Could you check a few things on this model? Use its own coordinates, in mm. A direction names the side the tool comes from. Round coordinates to 2 decimals unless told otherwise and drop trailing zeros. Loops run counter-clockwise (first coordinate to the right, second up) from the corner with the lowest first, then second, coordinate; pieces in that order, holes last. Notation, with made-up numbers: (-2.75, 64.25) -> (21.25, 64.25) arc R28 cw to (21.25, 83.25) -> close; hole circle Ø6 at (-28, -32). An arc over 180 degrees is marked (long way). One line per item, written item: value.
from build123d import *

# Parameters (mm, degrees)
F1_DEPTH = 11
F2_DEPTH = 4
F3_DEPTH = 10
F4_DEPTH = 5
F5_R     = 2


# Not quite as in the source:
# - a feature names something its author has since deleted; it is built from what else it names


with BuildPart() as f1:
    # F0 (on Top) → F1 (new body)
    with BuildSketch(Plane.XY):
        with BuildLine():
            ThreePointArc((93, 77.5), (92.267766953, 79.267766953), (90.5, 80))
            Line((90.5, 80), (37, 80))
            Line((37, 80), (25, 80))
            Line((25, 80), (19, 80))
            Line((19, 80), (-7, 80))
            Line((-7, 80), (-13, 80))
            Line((-13, 80), (-25, 80))
            Line((-25, 80), (-74, 80))
            Line((-74, 80), (-91.5, 80))
            ThreePointArc((-91.5, 80), (-93.267766953, 79.267766953), (-94, 77.5))
            Line((-94, 77.5), (-94, 76))
            Line((-94, 76), (-94, 0))
            Line((-94, 0), (-94, -1.5))
            ThreePointArc((-94, -1.5), (-93.267766953, -3.267766953), (-91.5, -4))
            Line((-91.5, -4), (-88, -4))
            Line((-88, -4), (-86, -4))
            Line((-86, -4), (-71, -4))
            Line((-71, -4), (-28.6959191337, -4))
            Line((-28.6959191337, -4), (67.7072161436, -4))
            Line((67.7072161436, -4), (88, -4))
            Line((88, -4), (90.5, -4))
            ThreePointArc((90.5, -4), (92.267766953, -3.267766953), (93, -1.5))
            Line((93, -1.5), (93, 0))
            Line((93, 0), (93, 76))
            Line((93, 76), (93, 77.5))
        make_face()
        with BuildLine():
            ThreePointArc((90, 2.5), (89.267766953, 0.732233047), (87.5, 0))
            Line((87.5, 0), (-87.5, 0))
            ThreePointArc((-87.5, 0), (-89.267766953, 0.732233047), (-90, 2.5))
            Line((-90, 2.5), (-90, 73.5))
            ThreePointArc((-90, 73.5), (-89.267766953, 75.267766953), (-87.5, 76))
            Line((-87.5, 76), (87.5, 76))
            ThreePointArc((87.5, 76), (89.267766953, 75.267766953), (90, 73.5))
            Line((90, 73.5), (90, 2.5))
        make_face(mode=Mode.SUBTRACT)
    extrude(amount=F1_DEPTH)

    # F0 (on Top) → F2 (join)
    with BuildSketch(Plane.XY):
        with BuildLine():
            Line((-87.5, 0), (87.5, 0))
            ThreePointArc((87.5, 0), (89.267766953, 0.732233047), (90, 2.5))
            Line((90, 2.5), (90, 73.5))
            ThreePointArc((90, 73.5), (89.267766953, 75.267766953), (87.5, 76))
            Line((87.5, 76), (-87.5, 76))
            ThreePointArc((-87.5, 76), (-89.267766953, 75.267766953), (-90, 73.5))
            Line((-90, 73.5), (-90, 2.5))
            ThreePointArc((-90, 2.5), (-89.267766953, 0.732233047), (-87.5, 0))
        make_face()
        with BuildLine():
            Line((-77.5, 66), (77.5, 66))
            ThreePointArc((77.5, 66), (79.267766953, 65.267766953), (80, 63.5))
            Line((80, 63.5), (80, 12.5))
            ThreePointArc((80, 12.5), (79.267766953, 10.732233047), (77.5, 10))
            Line((77.5, 10), (-77.5, 10))
            ThreePointArc((-77.5, 10), (-79.267766953, 10.732233047), (-80, 12.5))
            Line((-80, 12.5), (-80, 63.5))
            ThreePointArc((-80, 63.5), (-79.267766953, 65.267766953), (-77.5, 66))
        make_face(mode=Mode.SUBTRACT)
        with BuildLine():
            Line((-25, 80), (-13, 80))
            Line((-13, 80), (-13, 89.5))
            ThreePointArc((-13, 89.5), (-13.732233047, 91.267766953), (-15.5, 92))
            Line((-15.5, 92), (-22.5, 92))
            ThreePointArc((-22.5, 92), (-24.267766953, 91.267766953), (-25, 89.5))
            Line((-25, 89.5), (-25, 80))
        make_face()
        with BuildLine():
            Line((-7, 80), (19, 80))
            Line((19, 80), (19, 89.5))
            ThreePointArc((19, 89.5), (18.267766953, 91.267766953), (16.5, 92))
            Line((16.5, 92), (-4.5, 92))
            ThreePointArc((-4.5, 92), (-6.267766953, 91.267766953), (-7, 89.5))
            Line((-7, 89.5), (-7, 80))
        make_face()
        with BuildLine():
            Line((25, 80), (37, 80))
            Line((37, 80), (37, 89.5))
            ThreePointArc((37, 89.5), (36.267766953, 91.267766953), (34.5, 92))
            Line((34.5, 92), (27.5, 92))
            ThreePointArc((27.5, 92), (25.732233047, 91.267766953), (25, 89.5))
            Line((25, 89.5), (25, 80))
        make_face()
    extrude(amount=F2_DEPTH)

    # F0 (on Top) → F3 (join)
    with BuildSketch(Plane.XY):
        with BuildLine():
            Line((93, -81.5), (93, -1.5))
            ThreePointArc((93, -1.5), (92.267766953, -3.267766953), (90.5, -4))
            Line((90.5, -4), (88, -4))
            Line((88, -4), (67.7072161436, -4))
            ThreePointArc((67.7072161436, -4), (74.7782839555, -6.9289321881), (77.7072161436, -14))
            Line((77.7072161436, -14), (77.7072161436, -58.7379819401))
            ThreePointArc((77.7072161436, -58.7379819401), (73.0879609173, -67.1669549309), (63.4976990076, -67.8088124137))
            Line((63.4976990076, -67.8088124137), (-32.9054362697, -23.0708304737))
            ThreePointArc((-32.9054362697, -23.0708304737), (-38.4608642113, -11.8445771571), (-28.6959191337, -4))
            Line((-28.6959191337, -4), (-71, -4))
            Line((-71, -4), (-71, -10.9733034172))
            Line((-71, -10.9733034172), (-64.3552474564, -14.0623617917))
            Line((-64.3552474564, -14.0623617917), (80.7072161436, -81.5))
            Line((80.7072161436, -81.5), (93, -81.5))
        make_face()
    extrude(amount=F3_DEPTH)

    # F0 (on Top) → F4 (join)
    with BuildSketch(Plane.XY):
        Polygon((-71, -14.0623617917), (-71, -10.9733034172), (-86, -4), (-86, -14.0623617917), align=None)
        Polygon((-86, -4), (-71, -10.9733034172), (-71, -4), align=None)
        Polygon((-71, -14.0623617917), (-64.3552474564, -14.0623617917), (-71, -10.9733034172), align=None)
    extrude(amount=F4_DEPTH)

    # F5
    f5_edges = [f1.edges().sort_by_distance(p)[0] for p in [
        (86.853608, -81.5, 10),
    ]]
    fillet(f5_edges, radius=F5_R)


solid = f1.part
(1) Thinking about a two-plate mould opening in X: for faces 6 (the face through (-1, 66, 2)), 7 (the face through (6, 6, 0)), 8 (the face through (37, 85, 2)), which applies, released by +X, released by -X, zero draft, split by the parting line, or undercut?
Recorded:
face 6: undercut
face 7: zero draft
face 8: released by +X
(2) If we section it at D-D, the plane x = 70.5: Please give me the cut outline in (y, z).
Recorded:
outline: (-76.75, 0) -> (-68.34, 0) -> (-68.34, 10) -> (-76.75, 10) -> close; (-4.4, 0) -> (10, 0) -> (10, 4) -> (0, 4) -> (0, 11) -> (-4, 11) -> (-4, 10) -> (-4.4, 10) -> close; (66, 0) -> (80, 0) -> (80, 11) -> (76, 11) -> (76, 4) -> (66, 4) -> close
(3) I'm going to push flat-ended pins straight in: pin 1 Ø2 at (x, z) = (-29, 6) entering from -Y; pin 2 Ø1 at (x, z) = (-19.5, 9.5) entering from -Y; pin 3 Ø5.5 at (y, z) = (-7.5, 1.5) entering from -X. Where does each tip first touch, or does it pass through?
Recorded:
pin 1: y = -30.96
pin 2: y = -35.15
pin 3: x = -86
(4) If I drill on L1, parallel to X at y = 59.5, z = 8; L2, parallel to Y at x = -79, z = 6.25; L3, parallel to Y at x = 10.5, z = 7.25, over which ranges is the centre line in solid material (lowest first)?
Recorded:
L1: -94 to -90, 90 to 93
L2: -4 to 0, 76 to 80
L3: -48.86 to -43.21, -4 to 0, 76 to 80
(5) If we section it at A-A, the plane y = 19.5: Please give me the cut outline in (x, z).
Recorded:
outline: (-94, 0) -> (-80, 0) -> (-80, 4) -> (-90, 4) -> (-90, 11) -> (-94, 11) -> close; (80, 0) -> (93, 0) -> (93, 11) -> (90, 11) -> (90, 4) -> (80, 4) -> close
(6) For faces 1 (the face through (-0.4, 66.3, 4)), 2 (the face through (-7, 85, 2)), 3 (the face through (-19, 86, 4)), 4 (the face through (80, 38, 2)), 5 (the face through (-75, -14.062, 2)), which set-ups out of +Z, -Z, +X, -X, +Y, -Y let a thin tool reach every point of the face, with its end or its side?
Recorded:
face 1: +Z
face 2: +Z, -Z, +Y
face 3: +Z, +X, -X, +Y
face 4: +Z, -Z
face 5: +Z, -Z, -X, -Y
(7) If we section it at B-B, the plane x = 10: Please give me the cut outline in (y, z).
Recorded:
outline: (-48.63, 0) -> (-42.98, 0) -> (-42.98, 10) -> (-48.63, 10) -> close; (-4, 0) -> (10, 0) -> (10, 4) -> (0, 4) -> (0, 11) -> (-4, 11) -> close; (66, 0) -> (92, 0) -> (92, 4) -> (80, 4) -> (80, 11) -> (76, 11) -> (76, 4) -> (66, 4) -> close
(8) If we section it at C-C, the plane y = -30.5: Please give me the cut outline in (x, z), then the cut area to 3 significant figures.
Recorded:
outline: (-29, 0) -> (-16.9, 0) -> (-16.9, 10) -> (-29, 10) -> close; (77.71, 0) -> (93, 0) -> (93, 10) -> (77.71, 10) -> close
area: 274 mm²
